```python
from build123d import *

# Parameters (mm, degrees)
F0_R     = 76.2
F0_R_2   = 38.1
F1_DEPTH = 25.4
F2_R     = 152.4
F2_R_2   = 76.2
F3_DEPTH = 100
F4_R     = 76.2
F4_R_2   = 38.1
F5_DEPTH = 100


with BuildPart() as f1:
    # F0 (on Top) → F1 (new body)
    with BuildSketch(Plane.XY):
        with BuildLine():
            ThreePointArc((101.056902, -114.075688), (138.972716, -62.548734), (152.4, 0))
            ThreePointArc((152.4, 0), (89.079536, 123.655151), (-48.263993, 144.555688))
            ThreePointArc((-48.263993, 144.555688), (-131.982272, -76.2), (101.056902, -114.075688))
        make_face()
        Circle(F0_R, mode=Mode.SUBTRACT)
        with BuildLine():
            ThreePointArc((-48.263993, 144.555688), (89.079536, 123.655151), (152.4, 0))
            ThreePointArc((152.4, 0), (138.972716, -62.548734), (101.056902, -114.075688))
            Line((101.056902, -114.075688), (380.48413, 133.462156))
            ThreePointArc((380.48413, 133.462156), (263.964543, 152.4), (305.823682, 262.777844))
            Line((305.823682, 262.777844), (-48.263993, 144.555688))
        make_face()
        with BuildLine():
            ThreePointArc((406.155679, 190.5), (374.495447, 252.327575), (305.823682, 262.777844))
            ThreePointArc((305.823682, 262.777844), (263.964543, 152.4), (380.48413, 133.462156))
            ThreePointArc((380.48413, 133.462156), (399.442037, 159.225633), (406.155679, 190.5))
        make_face()
        with Locations((329.955679, 190.5)):
            Circle(F0_R_2, mode=Mode.SUBTRACT)
    extrude(amount=F1_DEPTH)

    # F2 (on face) → F3 (join)
    with BuildSketch(Plane.XY.offset(25.4)):
        Circle(F2_R)
        Circle(F2_R_2, mode=Mode.SUBTRACT)
    extrude(amount=F3_DEPTH)

    # F4 (on face) → F5 (join, through all)
    with BuildSketch(Plane.XY.offset(25.4)):
        with Locations((329.955679, 190.5)):
            Circle(F4_R)
        with Locations((329.955679, 190.5)):
            Circle(F4_R_2, mode=Mode.SUBTRACT)
    extrude(amount=F5_DEPTH)


solid = f1.part
```
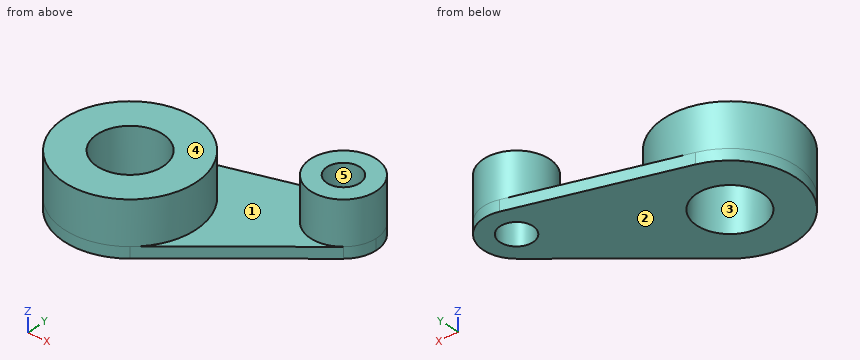
Check sheet for the modelled part. Datum: model origin and axes. Units: mm. Face numbers are marked on the shaded views. A direction names the side the tool comes from. Round coordinates to 2 decimals unless told otherwise and drop trailing zeros. Loops run counter-clockwise (first coordinate to the right, second up) from the corner with the lowest first, then second, coordinate; pieces in that order, holes last. Notation, with made-up numbers: (56, 38) - (108, 38) arc R12 ccw to (108, 42) - close; hole circle Ø5 at (-23.5, -8.75). An arc over 180 degrees is marked (long way). Answer as a JSON object with one key per item and string values. Group by question number.
Q1. Scan lines: line 1 along Y through (x, z) = (0, 81); line 2 along Z through (x, y) = (245, 172); line 3 along X through (y, z) = (24, 61). Record each from-to range of solid material in increasing order. Write a range as [from, to].
Q2. Sectioned sample at D-D, the plane y = 0. Enter the section's corners in (x, z), plus the area to 3 significant figures.
Q3. Set-up check for the marked faces 1 and 2: record each of +Z, -Z, +X, -X, +Y, -Y from which the full face is reachable in a straight line by a thin tool's end or side.
Q4. Gauge pin test, flat ends, axial feed: P1, Ø1.5, axis at y = 128.5, z = 89.5, coming from the -X side; P2, Ø1.5, axis at y = 170, z = 44, coming from the +X side; P3, Ø5, axis at x = -77.5, z = 67, coming from the +Y side. Record the tip position at first contact, or that the pin passes through.
Q5. Sectioned sample at A-A, the plane z = 14.5. Enter the section's corners in (x, y).
Q6. Sectioned sample at B-B, the plane z = 40. Enter the section's corners in (x, y).
Q7. Sectioned sample at C-C, the plane x = 0. Enter the section's corners in (y, z), plus the area to 3 significant figures.
Q8. Mould release check, pull along X, two halves, no side actions. Record for the marked faces 3, 4 and 5: released by +X, released by -X, zero draft, split by the parting line, or undercut.
Solution:
{
 "1": {"line 1": "y = [-152.4, -76.2], [76.2, 152.4]", "line 2": "z = [0, 25.4]", "line 3": "x = [-150.5, -72.32], [72.32, 150.5]"},
 "2": {"outline": "(-152.4, 0) - (-76.2, 0) - (-76.2, 125.4) - (-152.4, 125.4) - close; (76.2, 0) - (229.83, 0) - (229.83, 25.4) - (152.4, 25.4) - (152.4, 125.4) - (76.2, 125.4) - close", "area": "21,100 mm²"},
 "3": {"face 1": "+Z", "face 2": "-Z, +X, -X, +Y, -Y"},
 "4": {"P1": "stops at x = -83.1", "P2": "stops at x = 403.55", "P3": "stops at y = 132.67"},
 "5": {"outline": "(-48.26, 144.56) arc R152.4 ccw (long way) to (101.06, -114.08) - (380.48, 133.46) arc R76.2 ccw to (406.16, 190.5) arc R76.2 ccw to (305.82, 262.78) - close; hole circle Ø152.4 at (0, 0); hole circle Ø76.2 at (329.96, 190.5)"},
 "6": {"outline": "circle Ø304.8 at (0, 0); circle Ø152.4 at (329.96, 190.5); hole circle Ø152.4 at (0, 0); hole circle Ø76.2 at (329.96, 190.5)"},
 "7": {"outline": "(-152.4, 0) - (-76.2, 0) - (-76.2, 125.4) - (-152.4, 125.4) - close; (76.2, 0) - (160.67, 0) - (160.67, 25.4) - (152.4, 25.4) - (152.4, 125.4) - (76.2, 125.4) - close", "area": "19,300 mm²"},
 "8": {"face 3": "undercut", "face 4": "zero draft", "face 5": "undercut"}
}
